```python
from build123d import *

# Parameters (mm, degrees)
SKETCH_2_W                 = 240.549430728
SKETCH_2_H                 = 149.540933388
EXTRUDE_1_DEPTH            = 5
SKETCH_6_W                 = 93.246571425
SKETCH_6_H                 = 149.540933388
EXTRUDE_4_DEPTH            = 5
SKETCH_8_W                 = 274.716709757
SKETCH_8_H                 = 58.51354913
EXTRUDE_6_DEPTH            = 5
CUT_EXTRUDE_2_DEPTH        = 252.755772101
CUT_EXTRUDE_2_DEPTH_BACK   = 252.755772101
SKETCH_9_W                 = 59.079292396
SKETCH_9_H                 = 149.540933388
SKETCH_10_W                = 104.703380117
SKETCH_10_H                = 208.054482518
CUT_EXTRUDE_3_DEPTH        = 10
SKETCH_12_W                = 200
SKETCH_12_H                = 200
EXTRUDE_7_DEPTH            = 5
SKETCH_13_OUTSIDE_W        = 259.728
SKETCH_13_OUTSIDE_H        = 267.782
SKETCH_13_OUTSIDE_W_2      = 200
SKETCH_13_OUTSIDE_H_2      = 200
CUT_EXTRUDE_4_DEPTH        = 278.64321362
EXTRUDE_START              = -75
SKETCH_18_R                = 5.25
EXTRUDE_9_DEPTH            = 10
EXTRUDE_START_2            = -46
EXTRUDE_10_DEPTH           = 15
EXTRUDE_START_3            = -91.2
EXTRUDE_11_DEPTH           = 15
EXTRUDE_12_REACH           = 307.894
SKETCH_20_R                = 5.25
SKETCH_26_W                = 200
SKETCH_26_H                = 5
EXTRUDE_13_DEPTH           = 100
SKETCH_27_W                = 200
SKETCH_27_H                = 5
CUT_EXTRUDE_5_DEPTH        = 30
EXTRUDE_14_DEPTH           = 10
SKETCH_29_W                = 60
SKETCH_29_H                = 9
EXTRUDE_15_DEPTH           = 10
HOLE_WIZARD_M4_1_OUTLINE_R = 1.65
HOLE_WIZARD_M4_1_DEPTH     = 14
HOLE_WIZARD_M4_2_D         = 3.3
HOLE_START                 = -37.990466694
HOLE_WIZARD_M4_3_OUTLINE_R = 1.65
HOLE_WIZARD_M4_3_DEPTH     = 32
EXTRUDE_16_DEPTH           = 10
SKETCH_37_W                = 60
SKETCH_37_H                = 9
EXTRUDE_17_DEPTH           = 10
HOLE_WIZARD_M4_4_OUTLINE_R = 1.65
HOLE_WIZARD_M4_4_DEPTH     = 14
EXTRUDE_START_4            = -3.5
SKETCH_40_R                = 5.25
SKETCH_40_R_2              = 3.25
EXTRUDE_18_DEPTH           = 46.5
CUT_EXTRUDE_START          = -3.5
SKETCH_41_R                = 5.25
SKETCH_41_R_2              = 3.25
CUT_EXTRUDE_6_DEPTH        = 3.5
HOLE_WIZARD_M4_5_OUTLINE_R = 1.65
HOLE_WIZARD_M4_5_DEPTH     = 14


# Read off the part's stored shape, not the designer's step: M4 螺纹孔1, M4 螺纹孔3, M4 螺纹孔4, M4 螺纹孔5
with BuildPart() as part:
    # 草图2 → 凸台-拉伸1 (new body)
    with BuildSketch(Plane(origin=(0, 0, 0), x_dir=(1, 0, 0), z_dir=(0, 1, 0))):
        Rectangle(SKETCH_2_W, SKETCH_2_H)
    extrude(amount=EXTRUDE_1_DEPTH)

    # 草图6 → 凸台-拉伸4 (add)
    with BuildSketch(Plane(origin=(0, 5, 0), x_dir=(1, 0, 0), z_dir=(0, 1, 0))):
        with Locations((166.898001077, 0)):
            Rectangle(SKETCH_6_W, SKETCH_6_H)
    extrude(amount=-EXTRUDE_4_DEPTH)

    # 草图8 → 凸台-拉伸6 (add)
    with BuildSketch(Plane(origin=(0, 5, 0), x_dir=(1, 0, 0), z_dir=(0, 1, 0))):
        with Locations((76.162931911, -104.027241259)):
            Rectangle(SKETCH_8_W, SKETCH_8_H)
    extrude(amount=-EXTRUDE_6_DEPTH)

    # 草图9 → 切除-拉伸2 (cut, two sides: drawn at the far end of the back side and taken through both)
    with BuildSketch(Plane(origin=(0, 5, 0), x_dir=(1, 0, 0), z_dir=(0, 1, 0)).offset(-CUT_EXTRUDE_2_DEPTH_BACK)):
        with Locations((-90.735069166, 0)):
            Rectangle(SKETCH_9_W, SKETCH_9_H)
    extrude(amount=CUT_EXTRUDE_2_DEPTH + CUT_EXTRUDE_2_DEPTH_BACK, mode=Mode.SUBTRACT)

    # 草图10 → 切除-拉伸3 (cut)
    with BuildSketch(Plane(origin=(0, 5, 0), x_dir=(1, 0, 0), z_dir=(0, 1, 0))):
        with Locations((-8.84373291, -29.256774565)):
            Rectangle(SKETCH_10_W, SKETCH_10_H)
    extrude(amount=-CUT_EXTRUDE_3_DEPTH, mode=Mode.SUBTRACT)

    # 草图12 → 凸台-拉伸7 (add)
    with BuildSketch(Plane(origin=(0, 5, 0), x_dir=(1, 0, 0), z_dir=(0, 1, 0))):
        with Locations((143.507957149, -25.229533306)):
            Rectangle(SKETCH_12_W, SKETCH_12_H)
    extrude(amount=-EXTRUDE_7_DEPTH)

    # 草图13 outside → 切除-拉伸4 (cut, through all)
    with BuildSketch(Plane(origin=(0, 5, 0), x_dir=(1, 0, 0), z_dir=(0, 1, 0))):
        with Locations((143.508, -29.257)):
            Rectangle(SKETCH_13_OUTSIDE_W, SKETCH_13_OUTSIDE_H)
        with Locations((143.507957149, -25.229533306)):
            Rectangle(SKETCH_13_OUTSIDE_W_2, SKETCH_13_OUTSIDE_H_2, mode=Mode.SUBTRACT)
    extrude(amount=-CUT_EXTRUDE_4_DEPTH, mode=Mode.SUBTRACT)

    # 草图18 → 凸台-拉伸9 (add)
    with BuildSketch(Plane.XY.offset(125.229533306).offset(EXTRUDE_START)):
        with BuildLine():
            Line((95.507957149, 14), (95.507957149, 125))
            ThreePointArc((95.507957149, 125), (88.507957149, 132), (81.507957149, 125))
            Line((81.507957149, 125), (81.507957149, 14))
            Line((81.507957149, 14), (68.507957149, 14))
            Line((68.507957149, 14), (68.507957149, 5))
            Line((68.507957149, 5), (108.507957149, 5))
            Line((108.507957149, 5), (108.507957149, 14))
            Line((108.507957149, 14), (95.507957149, 14))
        make_face()
        with Locations((88.507957149, 125)):
            Circle(SKETCH_18_R, mode=Mode.SUBTRACT)
    extrude_9 = extrude(amount=-EXTRUDE_9_DEPTH)

    # 镜向1: 凸台-拉伸9 across plane
    add(extrude_9.mirror(Plane.XY.offset(25.229533306)))

    # 草图16 → 凸台-拉伸10 (add)
    with BuildSketch(Plane(origin=(243.507957149, 0, 0), x_dir=(0, 0, -1), z_dir=(1, 0, 0)).offset(EXTRUDE_START_2)):
        with BuildLine():
            Line((-53.779533306, 14), (-53.779533306, 145.085631965))
            Line((-53.779533306, 145.085631965), (-67.779533306, 145.085631965))
            Line((-67.779533306, 145.085631965), (-67.779533306, 139.085631965))
            ThreePointArc((-67.779533306, 139.085631965), (-69.779533306, 114.75), (-71.779533306, 139.085631965))
            Line((-71.779533306, 139.085631965), (-71.779533306, 145.085631965))
            Line((-71.779533306, 145.085631965), (-85.779533306, 145.085631965))
            Line((-85.779533306, 145.085631965), (-85.779533306, 14))
            Line((-85.779533306, 14), (-99.779533306, 14))
            Line((-99.779533306, 14), (-99.779533306, 5))
            Line((-99.779533306, 5), (-39.779533306, 5))
            Line((-39.779533306, 5), (-39.779533306, 14))
            Line((-39.779533306, 14), (-53.779533306, 14))
        make_face()
    extrude(amount=-EXTRUDE_10_DEPTH)

    # 草图19 → 凸台-拉伸11 (add)
    with BuildSketch(Plane(origin=(243.507957149, 0, 0), x_dir=(0, 0, -1), z_dir=(1, 0, 0)).offset(EXTRUDE_START_3)):
        with BuildLine():
            Line((37.990466694, 14), (37.990466694, 144.933566106))
            Line((37.990466694, 144.933566106), (23.990466694, 144.933566106))
            Line((23.990466694, 144.933566106), (23.990466694, 138.933566106))
            ThreePointArc((23.990466694, 138.933566106), (21.990466694, 114.9), (19.990466694, 138.933566106))
            Line((19.990466694, 138.933566106), (19.990466694, 144.933566106))
            Line((19.990466694, 144.933566106), (5.990466694, 144.933566106))
            Line((5.990466694, 144.933566106), (5.990466694, 14))
            Line((5.990466694, 14), (-8.009533306, 14))
            Line((-8.009533306, 14), (-8.009533306, 5))
            Line((-8.009533306, 5), (51.990466694, 5))
            Line((51.990466694, 5), (51.990466694, 14))
            Line((51.990466694, 14), (37.990466694, 14))
        make_face()
    extrude(amount=-EXTRUDE_11_DEPTH)

    # 草图20 → 凸台-拉伸12 (add, up to next)
    with BuildSketch(Plane(origin=(0, 0, 40.229533306), x_dir=(-1, 0, 0), z_dir=(0, 0, -1)), mode=Mode.PRIVATE) as extrude_12_sk1:
        with BuildLine():
            Line((-108.507957149, 5), (-68.507957149, 5))
            Line((-68.507957149, 5), (-68.507957149, 14))
            Line((-68.507957149, 14), (-81.507957149, 14))
            Line((-81.507957149, 14), (-81.507957149, 125))
            ThreePointArc((-81.507957149, 125), (-88.507957149, 132), (-95.507957149, 125))
            Line((-95.507957149, 125), (-95.507957149, 14))
            Line((-95.507957149, 14), (-108.507957149, 14))
            Line((-108.507957149, 14), (-108.507957149, 5))
        make_face()
        with Locations(Location((-88.507957149, 125, 0), (0, 0, 180))):
            Circle(SKETCH_20_R, mode=Mode.SUBTRACT)
    extrude_12_tool1 = extrude(extrude_12_sk1.sketch, amount=EXTRUDE_12_REACH, mode=Mode.PRIVATE) - part.part
    add(extrude_12_tool1.solids().sort_by_distance((88.507957, 57.997401, 40.229533))[0])

    # 草图26 → 凸台-拉伸13 (add)
    with BuildSketch(Plane(origin=(243.507957149, 0, 0), x_dir=(0, 0, -1), z_dir=(1, 0, 0))):
        with Locations((-25.229533306, 2.5)):
            Rectangle(SKETCH_26_W, SKETCH_26_H)
    extrude(amount=EXTRUDE_13_DEPTH)

    # 草图27 → 切除-拉伸5 (cut)
    with BuildSketch(Plane(origin=(343.507957149, 0, 0), x_dir=(0, 0, -1), z_dir=(1, 0, 0))):
        with Locations((-25.229533306, 2.5)):
            Rectangle(SKETCH_27_W, SKETCH_27_H)
    extrude(amount=-CUT_EXTRUDE_5_DEPTH, mode=Mode.SUBTRACT)

    # 草图28 → 凸台-拉伸14 (add)
    with BuildSketch(Plane(origin=(197.507957149, 0, 0), x_dir=(0, 0, -1), z_dir=(1, 0, 0))):
        Polygon((-85.779533306, 14), (-53.779533306, 14), (-39.779533306, 14), (-39.779533306, 5), (-99.779533306, 5), (-99.779533306, 14), align=None)
    extrude(amount=EXTRUDE_14_DEPTH)

    # 草图29 → 凸台-拉伸15 (add)
    with BuildSketch(Plane.ZY.offset(-182.507957149)):
        with Locations((69.779533306, 9.5)):
            Rectangle(SKETCH_29_W, SKETCH_29_H)
    extrude(amount=EXTRUDE_15_DEPTH)

    # M4 螺纹孔1 outline → M4 螺纹孔1 (cut)
    with BuildSketch(Plane(origin=(0, 0, 0), x_dir=(1, 0, 0), z_dir=(0, 1, 0))):
        with Locations((178.507957149, -91.779533306)):
            Circle(HOLE_WIZARD_M4_1_OUTLINE_R)
        with Locations((201.507957149, -91.779533306)):
            Circle(HOLE_WIZARD_M4_1_OUTLINE_R)
        with Locations((201.507957149, -47.779533306)):
            Circle(HOLE_WIZARD_M4_1_OUTLINE_R)
        with Locations((178.507957149, -47.779533306)):
            Circle(HOLE_WIZARD_M4_1_OUTLINE_R)
    extrude(amount=HOLE_WIZARD_M4_1_DEPTH, mode=Mode.SUBTRACT)

    # M4 螺纹孔2 (through all)
    with Locations(Plane.XY.offset(85.779533306)):
        with Locations((190.007957149, 141.085631965)):
            Hole(HOLE_WIZARD_M4_2_D / 2)

    # M4 螺纹孔3 outline → M4 螺纹孔3 (cut)
    with BuildSketch(Plane.XY.offset(HOLE_START)):
        with Locations((144.807957149, 140.933566106)):
            Circle(HOLE_WIZARD_M4_3_OUTLINE_R)
    extrude(amount=HOLE_WIZARD_M4_3_DEPTH, mode=Mode.SUBTRACT)

    # 草图36 → 凸台-拉伸16 (add)
    with BuildSketch(Plane(origin=(152.307957149, 0, 0), x_dir=(0, 0, -1), z_dir=(1, 0, 0))):
        Polygon((5.990466694, 14), (37.990466694, 14), (51.990466694, 14), (51.990466694, 5), (-8.009533306, 5), (-8.009533306, 14), align=None)
    extrude(amount=EXTRUDE_16_DEPTH)

    # 草图37 → 凸台-拉伸17 (add)
    with BuildSketch(Plane.ZY.offset(-137.307957149)):
        with Locations((-21.990466694, 9.5)):
            Rectangle(SKETCH_37_W, SKETCH_37_H)
    extrude(amount=EXTRUDE_17_DEPTH)

    # M4 螺纹孔4 outline → M4 螺纹孔4 (cut)
    with BuildSketch(Plane(origin=(0, 0, 0), x_dir=(1, 0, 0), z_dir=(0, 1, 0))):
        with Locations((133.307957149, -0.009533306)):
            Circle(HOLE_WIZARD_M4_4_OUTLINE_R)
        with Locations((156.307957149, -0.009533306)):
            Circle(HOLE_WIZARD_M4_4_OUTLINE_R)
        with Locations((156.307957149, 43.990466694)):
            Circle(HOLE_WIZARD_M4_4_OUTLINE_R)
        with Locations((133.307957149, 43.990466694)):
            Circle(HOLE_WIZARD_M4_4_OUTLINE_R)
    extrude(amount=HOLE_WIZARD_M4_4_DEPTH, mode=Mode.SUBTRACT)

    # 草图40 → 凸台-拉伸18 (add)
    with BuildSketch(Plane.XY.offset(50.229533306).offset(EXTRUDE_START_4)):
        with Locations((88.507957149, 125)):
            Circle(SKETCH_40_R)
        with Locations((88.507957149, 125)):
            Circle(SKETCH_40_R_2, mode=Mode.SUBTRACT)
    extrude(amount=-EXTRUDE_18_DEPTH)

    # 草图41 → 切除-拉伸6 (cut)
    with BuildSketch(Plane(origin=(0, 0, 0.229533306), x_dir=(-1, 0, 0), z_dir=(0, 0, -1)).offset(CUT_EXTRUDE_START)):
        with Locations(Location((-88.507957149, 125, 0), (0, 0, 180))):
            Circle(SKETCH_41_R)
        with Locations(Location((-88.507957149, 125, 0), (0, 0, 180))):
            Circle(SKETCH_41_R_2, mode=Mode.SUBTRACT)
    extrude(amount=CUT_EXTRUDE_6_DEPTH, mode=Mode.SUBTRACT)

    # M4 螺纹孔5 outline → M4 螺纹孔5 (cut)
    with BuildSketch(Plane(origin=(0, 0, 0), x_dir=(1, 0, 0), z_dir=(0, 1, 0))):
        with Locations((73.507957149, -42.229533306)):
            Circle(HOLE_WIZARD_M4_5_OUTLINE_R)
        with Locations((103.507957149, -42.229533306)):
            Circle(HOLE_WIZARD_M4_5_OUTLINE_R)
        with Locations((103.507957149, -8.229533306)):
            Circle(HOLE_WIZARD_M4_5_OUTLINE_R)
        with Locations((73.507957149, -8.229533306)):
            Circle(HOLE_WIZARD_M4_5_OUTLINE_R)
    extrude(amount=HOLE_WIZARD_M4_5_DEPTH, mode=Mode.SUBTRACT)


solid = part.part
```
Input: part model. Units: mm. Frame: model coordinates. A direction names the side the tool comes from. Round coordinates to 2 decimals unless told otherwise and drop trailing zeros. Loops run counter-clockwise (first coordinate to the right, second up) from the corner with the lowest first, then second, coordinate; pieces in that order, holes last.
1) Section query B-B on z = 78.5. Return the cut outline in (x, y).
Ans:
outline: (43.51, 0) - (313.51, 0) - (313.51, 5) - (207.51, 5) - (207.51, 14) - (197.51, 14) - (197.51, 118.4) - (182.51, 118.4) - (182.51, 14) - (172.51, 14) - (172.51, 5) - (43.51, 5) - close; (182.51, 135.6) - (197.51, 135.6) - (197.51, 145.09) - (182.51, 145.09) - close; hole circle Ø3.3 at (190.01, 141.09)
2) Section query C-C on z = 29. Return the cut outline in (x, y), plus the area to 3 significant figures.
Ans:
outline: (43.51, 0) - (313.51, 0) - (313.51, 5) - (108.51, 5) - (108.51, 14) - (95.51, 14) - (95.51, 125) arc R7 ccw to (81.51, 125) - (81.51, 14) - (68.51, 14) - (68.51, 5) - (43.51, 5) - close; hole circle Ø6.5 at (88.51, 125)
area: 3,310 mm2
3) Set-up query: faces 5 (the flat face through (108.508, 10, 26)), 6 (the flat face through (137.308, 80, -22)), 7 (the flat face through (152.308, 80, -22)), 8 (the flat face through (145, 80, -5.99)), 9 (the flat face through (190, 143, 67.78)). Return all of +Z, -Z, +X, -X, +Y, -Y with unobstructed straight access to the full face (end or side cutting, diameter ignored); none if empty.
Ans:
face 5: +Z, -Z, +Y
face 6: +Z, -Z, -X, +Y
face 7: +Z, -Z, +X, +Y
face 8: +Z, +X, -X, +Y
face 9: +X, -X, +Y
4) Section query D-D on x = 61.5. Return the cut outline in (y, z), plus the area to 3 significant figures.
Ans:
outline: (0, -74.77) - (5, -74.77) - (5, 125.23) - (0, 125.23) - close
area: 1,000 mm2
5) Pin query (flat end, axial travel): pin 1 (5 mm diameter, centred on x = 187.5, y = 110.5, fed in from -Z); pin 2 (2.5 mm diameter, centred on x = 182.5, y = 10.5, fed in from -Z); pin 3 (25 mm diameter, centred on y = 67, z = 22, fed in from -X). Return the tip coordinate at first contact, or that it passes through.
Ans:
pin 1: stops at z = 53.78
pin 2: stops at z = 39.78
pin 3: stops at x = 81.51
6) Pull-direction query (Z, two-part tool) for faces 1 (the flat face through (190, 145.086, 79)), 2 (the flat face through (145, 143, -19.99)), 3 (the flat face through (190, 143, 71.78)), 4 (the flat face through (190, 9, 99.78)); classes: released by +Z, released by -Z, zero draft, split by the parting line, or undercut.
Ans:
face 1: zero draft
face 2: undercut
face 3: undercut
face 4: released by +Z
7) Material intervals for line 1 (Z direction, x = 191.5, y = 127); line 2 (Y direction, x = 214, z = 68); line 3 (X direction, y = 125, z = 2.8), sorted ascending.
Ans:
line 1: z = 53.78 to 57.53, 82.03 to 85.78
line 2: y = 0 to 5
line 3: x = 81.51 to 83.26, 93.76 to 95.51
8) Section query A-A on y = 32. Return the cut outline in (x, z), plus the area to 3 significant figures.
Ans:
outline: (81.51, 0.23) - (95.51, 0.23) - (95.51, 50.23) - (81.51, 50.23) - close; (137.31, -37.99) - (152.31, -37.99) - (152.31, -5.99) - (137.31, -5.99) - close; (182.51, 53.78) - (197.51, 53.78) - (197.51, 85.78) - (182.51, 85.78) - close
area: 1,660 mm2
